Build history of the part. All positions in model axes, mm. Face numbers are marked on the shaded views. Give positions to 0.01 mm unless a question says otherwise; leave off trailing zeros. Loops run counter-clockwise (first coordinate to the right, second up) from the corner with the lowest first, then second, coordinate; pieces in that order, holes last. Notation, with made-up numbers: M 72.5,40.25 L 89.5,40.25 A12 ccw 89.5,58.25 Z; hole C -6,28 d9. An arc over 180 degrees is marked long. Put each result on its own line as item: value.
```python
from build123d import *

# Parameters (mm, degrees)
F2_DEPTH = 12.7
F1_R     = 7.14375
F3_DEPTH = 6.35


with BuildPart() as f2:
    # F1 (on Top) → F2 (new body)
    with BuildSketch(Plane.XY):
        with BuildLine():
            ThreePointArc((57.15, 0), (61.2719466085, 4.2155230865), (62.7124900485, 9.9326826377))
            ThreePointArc((62.7124900485, 9.9326826377), (59.575752362, 14.9248720794), (54.3528799063, 17.6603212285))
            ThreePointArc((54.3528799063, 17.6603212285), (56.9704158142, 22.9432734815), (56.5737545789, 28.8257677314))
            ThreePointArc((56.5737545789, 28.8257677314), (52.0478683856, 32.6043167785), (46.2353212285, 33.5919271685))
            ThreePointArc((46.2353212285, 33.5919271685), (47.0922237837, 39.4251764129), (44.8971858387, 44.8971858387))
            ThreePointArc((44.8971858387, 44.8971858387), (39.4251764129, 47.0922237837), (33.5919271685, 46.2353212285))
            ThreePointArc((33.5919271685, 46.2353212285), (32.6043167785, 52.0478683856), (28.8257677314, 56.5737545789))
            ThreePointArc((28.8257677314, 56.5737545789), (22.9432734815, 56.9704158142), (17.6603212285, 54.3528799063))
            ThreePointArc((17.6603212285, 54.3528799063), (14.9248720794, 59.575752362), (9.9326826377, 62.7124900485))
            ThreePointArc((9.9326826377, 62.7124900485), (4.2155230865, 61.2719466085), (0, 57.15))
            ThreePointArc((0, 57.15), (-4.2155230865, 61.2719466085), (-9.9326826377, 62.7124900485))
            ThreePointArc((-9.9326826377, 62.7124900485), (-14.9248720794, 59.575752362), (-17.6603212285, 54.3528799063))
            ThreePointArc((-17.6603212285, 54.3528799063), (-22.9432734815, 56.9704158142), (-28.8257677314, 56.5737545789))
            ThreePointArc((-28.8257677314, 56.5737545789), (-32.6043167785, 52.0478683856), (-33.5919271685, 46.2353212285))
            ThreePointArc((-33.5919271685, 46.2353212285), (-39.4251764129, 47.0922237837), (-44.8971858387, 44.8971858387))
            ThreePointArc((-44.8971858387, 44.8971858387), (-47.0922237837, 39.4251764129), (-46.2353212285, 33.5919271685))
            ThreePointArc((-46.2353212285, 33.5919271685), (-52.0478683856, 32.6043167785), (-56.5737545789, 28.8257677314))
            ThreePointArc((-56.5737545789, 28.8257677314), (-56.9704158142, 22.9432734815), (-54.3528799063, 17.6603212285))
            ThreePointArc((-54.3528799063, 17.6603212285), (-59.575752362, 14.9248720794), (-62.7124900485, 9.9326826377))
            ThreePointArc((-62.7124900485, 9.9326826377), (-61.2719466085, 4.2155230865), (-57.15, 0))
            ThreePointArc((-57.15, 0), (-61.2719466085, -4.2155230865), (-62.7124900485, -9.9326826377))
            ThreePointArc((-62.7124900485, -9.9326826377), (-59.575752362, -14.9248720794), (-54.3528799063, -17.6603212285))
            ThreePointArc((-54.3528799063, -17.6603212285), (-56.9704158142, -22.9432734815), (-56.5737545789, -28.8257677314))
            ThreePointArc((-56.5737545789, -28.8257677314), (-52.0478683856, -32.6043167785), (-46.2353212285, -33.5919271685))
            ThreePointArc((-46.2353212285, -33.5919271685), (-47.0922237837, -39.4251764129), (-44.8971858387, -44.8971858387))
            ThreePointArc((-44.8971858387, -44.8971858387), (-39.4251764129, -47.0922237837), (-33.5919271685, -46.2353212285))
            ThreePointArc((-33.5919271685, -46.2353212285), (-32.6043167785, -52.0478683856), (-28.8257677314, -56.5737545789))
            ThreePointArc((-28.8257677314, -56.5737545789), (-22.9432734815, -56.9704158142), (-17.6603212285, -54.3528799063))
            ThreePointArc((-17.6603212285, -54.3528799063), (-14.9248720794, -59.575752362), (-9.9326826377, -62.7124900485))
            ThreePointArc((-9.9326826377, -62.7124900485), (-4.2155230865, -61.2719466085), (0, -57.15))
            ThreePointArc((0, -57.15), (4.2155230865, -61.2719466085), (9.9326826377, -62.7124900485))
            ThreePointArc((9.9326826377, -62.7124900485), (14.9248720794, -59.575752362), (17.6603212285, -54.3528799063))
            ThreePointArc((17.6603212285, -54.3528799063), (22.9432734815, -56.9704158142), (28.8257677314, -56.5737545789))
            ThreePointArc((28.8257677314, -56.5737545789), (32.6043167785, -52.0478683856), (33.5919271685, -46.2353212285))
            ThreePointArc((33.5919271685, -46.2353212285), (39.4251764129, -47.0922237837), (44.8971858387, -44.8971858387))
            ThreePointArc((44.8971858387, -44.8971858387), (47.0922237837, -39.4251764129), (46.2353212285, -33.5919271685))
            ThreePointArc((46.2353212285, -33.5919271685), (52.0478683856, -32.6043167785), (56.5737545789, -28.8257677314))
            ThreePointArc((56.5737545789, -28.8257677314), (56.9704158142, -22.9432734815), (54.3528799063, -17.6603212285))
            ThreePointArc((54.3528799063, -17.6603212285), (59.575752362, -14.9248720794), (62.7124900485, -9.9326826377))
            ThreePointArc((62.7124900485, -9.9326826377), (61.2719466085, -4.2155230865), (57.15, 0))
        make_face()
        Polygon((0, 10.9985226281), (9.525, 5.499261314), (9.525, -5.499261314), (0, -10.9985226281), (-9.525, -5.499261314), (-9.525, 5.499261314), align=None, mode=Mode.SUBTRACT)
    extrude(amount=F2_DEPTH)

    # F1 (on Top) → F3 (join)
    with BuildSketch(Plane.XY):
        Polygon((9.525, -5.499261314), (9.525, 5.499261314), (0, 10.9985226281), (-9.525, 5.499261314), (-9.525, -5.499261314), (0, -10.9985226281), align=None)
        Circle(F1_R, mode=Mode.SUBTRACT)
    extrude(amount=F3_DEPTH)


solid = f2.part
```
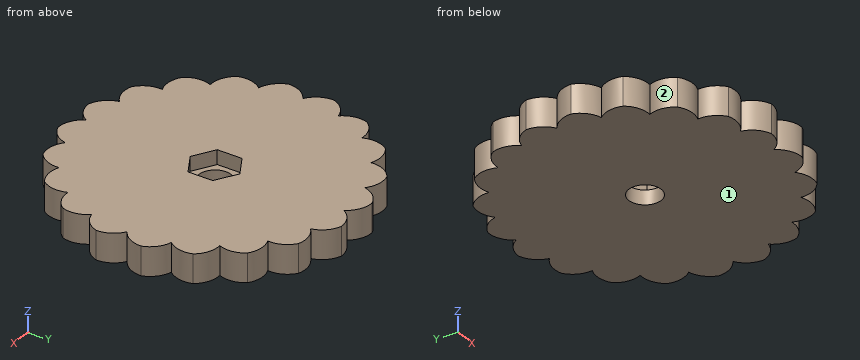
Q1. Drop flat-ended pins along their axis: pin 1 Ø7 at (y, z) = (0.5, 9.5) entering from -X; pin 2 Ø2 at (y, z) = (43, 2.5) entering from -X; pin 3 Ø4 at (x, z) = (-41.5, 9) entering from +Y; pin 4 Ø5.5 at (x, y) = (-3, -2) entering from +Z. Give the stop position or say it passes through.
Here are the results:
pin 1: x = -61.15
pin 2: x = -46.48
pin 3: y = 47.08
pin 4: through
Q2. Mould opens along Y. For the marked faces 1 and 2 say: pulls with the +Y half, pulls with the -Y half, needs draft (parallel to the pull), parting line crosses it, or undercut.
Here are the results:
face 1: needs draft
face 2: undercut
Q3. Slice it at A-A (x = 37.5). List the corners of the cut face in (y, z).
Here are the results:
outline: M -47.15,0 L 47.15,0 L 47.15,12.7 L -47.15,12.7 Z
Q4. Probe line 1 (Y direction, x = -26, z = 1.75); line 2 (Y direction, x = 55.5, z = 11); line 3 (Y direction, x = 38, z = 2). List the from-to ranges inside material, lowest first. Write a range as from..to.
Here are the results:
line 1: -57.16..57.16
line 2: -30.14..-19.21, -17.34..17.34, 19.21..30.14
line 3: -47.17..47.17
